Work out the finished part from the listing and answer in its coordinate system (mm). A direction names the side the tool comes from. Give positions to 0.01 mm unless a question says otherwise; leave off trailing zeros. Loops run counter-clockwise (first coordinate to the right, second up) from the corner with the lowest first, then second, coordinate; pieces in that order, holes last. Notation, with made-up numbers: (11, 40) - (21, 40) arc R14 ccw to (21, 61) - close; hole circle Ø3 at (84.25, 38). An arc over 180 degrees is marked (long way). One line per item, written item: value.
from build123d import *

# Parameters (mm, degrees)
BOSS_EXTRUDE1_DEPTH      = 20
SKETCH2_R                = 12.5
CUT_EXTRUDE1_DEPTH       = 7
SKETCH3_W                = 38
SKETCH3_H                = 15
CUT_EXTRUDE2_DEPTH       = 6
SKETCH7_W                = 30
SKETCH7_H                = 40
BOSS_EXTRUDE2_DEPTH      = 10
BOSS_EXTRUDE3_DEPTH      = 15
BOSS_EXTRUDE3_DEPTH_BACK = 45
SKETCH8_R                = 10


with BuildPart() as part:
    # Sketch1 → Boss-Extrude1 (new body)
    with BuildSketch(Plane(origin=(0, 0, 0), x_dir=(1, 0, 0), z_dir=(0, 1, 0))):
        Polygon((0, 0), (30, 0), (30, 150), (60, 150), (60, 200), (-30, 200), (-30, 150), (0, 150), align=None)
    extrude(amount=BOSS_EXTRUDE1_DEPTH)

    # Sketch2 → Cut-Extrude1 (cut)
    with BuildSketch(Plane(origin=(0, 20, 0), x_dir=(1, 0, 0), z_dir=(0, 1, 0))):
        with Locations(Location((15, 175, 0), (0, 0, 270))):
            Circle(SKETCH2_R)
    extrude(amount=-CUT_EXTRUDE1_DEPTH, mode=Mode.SUBTRACT)

    # Sketch3 → Cut-Extrude2 (cut)
    with BuildSketch(Plane(origin=(0, 20, 0), x_dir=(1, 0, 0), z_dir=(0, 1, 0))):
        with Locations((41, 175)):
            Rectangle(SKETCH3_W, SKETCH3_H)
    extrude(amount=-CUT_EXTRUDE2_DEPTH, mode=Mode.SUBTRACT)

    # Sketch7 → Boss-Extrude2 (add)
    with BuildSketch(Plane(origin=(0, 20, 0), x_dir=(1, 0, 0), z_dir=(0, 1, 0))):
        with Locations((15, 20)):
            Rectangle(SKETCH7_W, SKETCH7_H)
    extrude(amount=BOSS_EXTRUDE2_DEPTH)

    # Sketch8 → Boss-Extrude3 (add, two sides: drawn at the far end of the back side and taken through both)
    with BuildSketch(Plane(origin=(30, 0, 0), x_dir=(0, 0, -1), z_dir=(1, 0, 0)).offset(-BOSS_EXTRUDE3_DEPTH_BACK)):
        with Locations((20, 15)):
            Circle(SKETCH8_R)
    extrude(amount=BOSS_EXTRUDE3_DEPTH + BOSS_EXTRUDE3_DEPTH_BACK)


solid = part.part
1. The mould has two halves that part along Z. Classify faces 6 (the flat face through (-30, 10, -175)), 7 (the cylindrical face through (-7.6, 18, -29.54)), 8 (the flat face through (15, 15, 0)): released by +Z, released by -Z, zero draft, split by the parting line, or undercut.
Output:
face 6: zero draft
face 7: undercut
face 8: released by +Z
2. Flat-ended cylindrical pins translate along their axes: pin 1 Ø12 at (y, z) = (16, -90) entering from -X; pin 2 Ø16 at (x, y) = (-9, 9) entering from +Z; pin 3 Ø10 at (y, z) = (19, -21) entering from +X. Find the tip coordinate at first contact, or state that the pin passes through.
Output:
pin 1: stops at x = 0
pin 2: stops at z = -10
pin 3: stops at x = 45
3. Section D-D (x = 15) is taken. Write down the section's boundary in (y, z).
Output:
outline: (0, -200) - (20, -200) - (20, -187.5) - (13, -187.5) - (13, -162.5) - (20, -162.5) - (20, -40) - (30, -40) - (30, 0) - (0, 0) - close
4. For faces 1 (the flat face through (45, 15, -20)), 2 (the flat face through (42, 14, -175)), 3 (the cylindrical face through (2.797, 16.549, -177.71)), 4 (the flat face through (-15, 10, -150)), 5 (the flat face through (45, 10, -150)), determine the directions among +Z, -Z, +X, -X, +Y, -Y from which every point of the face is accessible in a straight line to the end or side of a thin tool.
Output:
face 1: +Z, +X, +Y, -Y
face 2: +X, +Y
face 3: +Y
face 4: -X, +Y, -Y
face 5: +X, +Y, -Y
5. Section B-B (z = -175) is taken. Write down the section's boundary in (x, y).
Output:
outline: (-30, 0) - (60, 0) - (60, 14) - (27.5, 14) - (27.5, 13) - (2.5, 13) - (2.5, 20) - (-30, 20) - close
6. Section C-C (y = 23) is taken. Write down the section's boundary in (x, z), and give its area (3 significant figures).
Output:
outline: (-15, -26) - (0, -26) - (0, -40) - (30, -40) - (30, -26) - (45, -26) - (45, -14) - (30, -14) - (30, 0) - (0, 0) - (0, -14) - (-15, -14) - close
area: 1,560 mm²
7. Section A-A (x = -9) is taken. Write down the section's boundary in (y, z), and give its area (3 significant figures).
Output:
outline: (0, -200) - (20, -200) - (20, -150) - (0, -150) - close; circle Ø20 at (15, -20)
area: 1,310 mm²
8. Find the intervals of material crossed by line 1 along Z through (x, y) = (15, 18.5); line 2 along Z through (x, y) = (-10, 15.25); line 3 along Z through (x, y) = (29, 21.5), in increasing order.
Output:
line 1: z = -200 to -187.5, -162.5 to 0
line 2: z = -200 to -150, -30 to -10
line 3: z = -40 to 0
